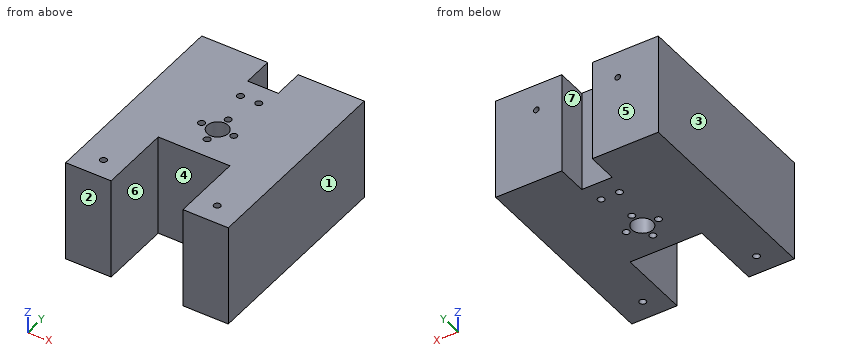
```python
from build123d import *

# Parameters (mm, degrees)
SKETCH_1_W           = 80
SKETCH_1_H           = 103.5
EXTRUDE_1_DEPTH      = 50
SKETCH_5_R           = 1.65
CUT_EXTRUDE_4_DEPTH  = 60
SKETCH_7_W           = 15
SKETCH_7_H           = 15
CUT_EXTRUDE_6_DEPTH  = 100
SKETCH_8_R           = 1.65
CUT_EXTRUDE_7_DEPTH  = 100
SKETCH_9_R           = 5.15
CUT_EXTRUDE_8_DEPTH  = 1000
SKETCH_10_W          = 80
SKETCH_10_H          = 1.5
CUT_EXTRUDE_9_DEPTH  = 10000
SKETCH_11_W          = 35.3
SKETCH_11_H          = 35.3
CUT_EXTRUDE_10_DEPTH = 1000
SKETCH_12_R          = 1.65
CUT_EXTRUDE_11_DEPTH = 1000
SKETCH_14_R          = 1.4
CUT_EXTRUDE_12_DEPTH = 35


with BuildPart() as part:
    # 草图1 → 凸台-拉伸1 (new body)
    with BuildSketch(Plane.XY):
        Rectangle(SKETCH_1_W, SKETCH_1_H)
    extrude(amount=EXTRUDE_1_DEPTH)

    # 草图5 → 切除-拉伸4 (cut)
    with BuildSketch(Plane.XY.offset(50)):
        with Locations((7.925, 2.75)):
            Circle(SKETCH_5_R)
        with Locations((-7.925, 2.75)):
            Circle(SKETCH_5_R)
        with Locations((0, 10.675)):
            Circle(SKETCH_5_R)
        with Locations((0, -5.175)):
            Circle(SKETCH_5_R)
    extrude(amount=-CUT_EXTRUDE_4_DEPTH, mode=Mode.SUBTRACT)

    # 草图7 → 切除-拉伸6 (cut)
    with BuildSketch(Plane.XY.offset(50)):
        with Locations((0, 44.25)):
            Rectangle(SKETCH_7_W, SKETCH_7_H)
    extrude(amount=-CUT_EXTRUDE_6_DEPTH, mode=Mode.SUBTRACT)

    # 草图8 → 切除-拉伸7 (cut)
    with BuildSketch(Plane.XY.offset(50)):
        with Locations((4.5, 26.75)):
            Circle(SKETCH_8_R)
        with Locations((-4.5, 26.75)):
            Circle(SKETCH_8_R)
    extrude(amount=-CUT_EXTRUDE_7_DEPTH, mode=Mode.SUBTRACT)

    # 草图9 → 切除-拉伸8 (cut)
    with BuildSketch(Plane.XY.offset(50)):
        with Locations((0, 2.75)):
            Circle(SKETCH_9_R)
    extrude(amount=-CUT_EXTRUDE_8_DEPTH, mode=Mode.SUBTRACT)

    # 草图10 → 切除-拉伸9 (cut)
    with BuildSketch(Plane.XY.offset(50)):
        with Locations((0, -51)):
            Rectangle(SKETCH_10_W, SKETCH_10_H)
    extrude(amount=-CUT_EXTRUDE_9_DEPTH, mode=Mode.SUBTRACT)

    # 草图11 → 切除-拉伸10 (cut)
    with BuildSketch(Plane.XY.offset(50)):
        with Locations((0, -32.6)):
            Rectangle(SKETCH_11_W, SKETCH_11_H)
    extrude(amount=-CUT_EXTRUDE_10_DEPTH, mode=Mode.SUBTRACT)

    # 草图12 → 切除-拉伸11 (cut)
    with BuildSketch(Plane.XY.offset(50)):
        with Locations((28, -40.25)):
            Circle(SKETCH_12_R)
        with Locations((-28, -40.25)):
            Circle(SKETCH_12_R)
    extrude(amount=-CUT_EXTRUDE_11_DEPTH, mode=Mode.SUBTRACT)

    # 草图14 → 切除-拉伸12 (cut)
    with BuildSketch(Plane(origin=(0, 51.75, 0), x_dir=(1, 0, 0), z_dir=(0, 1, 0))):
        with Locations(Location((20, -37, 0), (0, 0, 270))):
            Circle(SKETCH_14_R)
        with Locations(Location((-20, -37, 0), (0, 0, 270))):
            Circle(SKETCH_14_R)
    extrude(amount=-CUT_EXTRUDE_12_DEPTH, mode=Mode.SUBTRACT)


solid = part.part
```
Build history of the part. All positions in model axes, mm. Face numbers are marked on the shaded views. A direction names the side the tool comes from. Round coordinates to 2 decimals unless told otherwise and drop trailing zeros. Loops run counter-clockwise (first coordinate to the right, second up) from the corner with the lowest first, then second, coordinate; pieces in that order, holes last.
Item 1: Saw through at D-D (x = -20). List the corners of the cut face in (y, z).
Item 2: Pin check, flat tip, straight feed: P1, Ø3, axis at x = -4.5, y = 26.75, coming from the +Z side. Stop position of the tip, or through.
Item 3: Saw through at A-A (y = 26.75). List the corners of the cut face in (x, z).
Item 4: Saw through at C-C (z = 37). State how many separate pieces and enclosed holes the cut face has, then the cut area to 3 significant figures.
Item 5: Which spindle directions (+Z, -Z, +X, -X, +Y, -Y) get a long thin tool onto all of the face, cutting with end or side? Do the marked faces 5, 6 and 7. Say none if no direction does.
Item 6: Saw through at B-B (y = -32). List the corners of the cut face in (x, z).
Item 7: Two-plate mould, pull along X, no slides. Class the marked faces 1, 2, 3 and 4: released by +X, released by -X, zero draft, split by the parting line, or undercut.
Item 8: Drill centre lines: line 1 along X through (y, z) = (-40, 7); line 2 along X through (y, z) = (47, 29); line 3 along Y through (x, z) = (28, 16.5). Where is each one in solid material? Low to high.
Worked answers:
1. outline: (-50.25, 0) - (51.75, 0) - (51.75, 35.6) - (16.75, 35.6) - (16.75, 38.4) - (51.75, 38.4) - (51.75, 50) - (-50.25, 50) - close
2. P1: passes through
3. outline: (-40, 0) - (-6.15, 0) - (-6.15, 50) - (-40, 50) - close; (-2.85, 0) - (2.85, 0) - (2.85, 50) - (-2.85, 50) - close; (6.15, 0) - (40, 0) - (40, 50) - (6.15, 50) - close; hole circle Ø2.8 at (-20, 37); hole circle Ø2.8 at (20, 37)
4. separate pieces: 1
4. enclosed holes: 9
4. area: 6,340 mm2
5. face 5: +Z, -Z, +X, -X, +Y
5. face 6: +Z, -Z, -Y
5. face 7: +Z, -Z, +Y
6. outline: (-40, 0) - (-17.65, 0) - (-17.65, 50) - (-40, 50) - close; (17.65, 0) - (40, 0) - (40, 50) - (17.65, 50) - close
7. face 1: released by +X
7. face 2: zero draft
7. face 3: released by -X
7. face 4: undercut
8. line 1: x = -40 to -29.63, -26.37 to -17.65, 17.65 to 26.37, 29.63 to 40
8. line 2: x = -40 to -7.5, 7.5 to 40
8. line 3: y = -50.25 to -41.9, -38.6 to 51.75
